Answer from the drawing. Dimensions are ordinates in mm from the lowest x, y and z of the part. Round coordinates to 2 decimals unless told otherwise and drop trailing zeros. Write each loop counter-clockwise with the first axis right and the second up, starting at its lowest first coordinate (ties: lowest second). Pieces come first, ordered by that corner, then holes. Notation, with made-up numbers: (44, -15.75) -> (89, -15.75) arc R3 cw to (89, -10.75) -> close; hole circle Ø1 at (81.5, 62). An arc over 180 degrees is marked (long way). Answer as a JSON object with one key per item and string values. Group by question number.
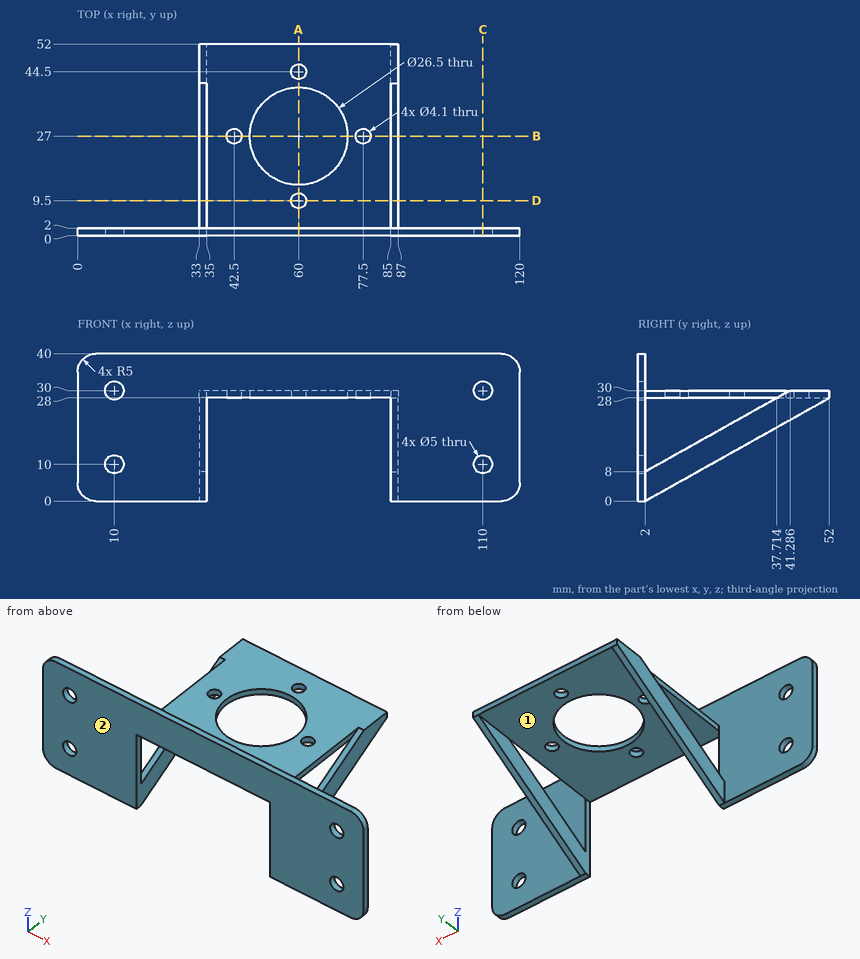
1) A cutting plane is placed at B-B on y = 27. Determine the outline of the cut face in (x, z).
2) Each of these flat-tipped pins is pushed along its axis until it touches: P1, Ø25, axis at x = 49, y = 29.5, coming from the +Z side; P2, Ø6, axis at y = 29, z = 29.5, coming from the +X side; P3, Ø22.5, axis at y = 31, z = 16, coming from the +X side; P4, Ø3.5, axis at x = 42.5, y = 27, coming from the +Z side. Where does it stop, or does it pass through?
3) Straight lines are drawn through the part: L1, parallel to X at y = 0.8, z = 10; L2, parallel to X at y = 0.5, z = 30; L3, parallel to Y at x = 42.5, z = 29.25. For each, find the intervals that lie inside material, in ascending order.
4) A cutting plane is placed at C-C on x = 110. Determine the outline of the cut face in (y, z), plus the area to 3 significant figures.
5) A cutting plane is placed at D-D on y = 9.5. Determine the outline of the cut face in (x, z).
6) A cutting plane is placed at A-A on x = 60. Determine the outline of the cut face in (y, z).
7) For a pull along X with two mould halves and no side action, classify the marked faces 1 and 2 as released by +X, released by -X, zero draft, split by the parting line, or undercut.
Established:
{
 "1": {"outline": "(33, 14) -> (35, 14) -> (35, 22) -> (33, 22) -> close; (35, 28) -> (40.45, 28) -> (40.45, 30) -> (35, 30) -> close; (44.55, 28) -> (46.75, 28) -> (46.75, 30) -> (44.55, 30) -> close; (73.25, 28) -> (75.45, 28) -> (75.45, 30) -> (73.25, 30) -> close; (79.55, 28) -> (85, 28) -> (85, 30) -> (79.55, 30) -> close; (85, 14) -> (87, 14) -> (87, 22) -> (85, 22) -> close"},
 "2": {"P1": "stops at z = 30", "P2": "stops at x = 85", "P3": "stops at x = 87", "P4": "passes through"},
 "3": {"L1": "x = 0 to 7.5, 12.5 to 35, 85 to 107.5, 112.5 to 120", "L2": "x = 0 to 7.5, 12.5 to 107.5, 112.5 to 120", "L3": "y = 0 to 24.95, 29.05 to 52"},
 "4": {"outline": "(0, 0) -> (2, 0) -> (2, 7.5) -> (0, 7.5) -> close; (0, 12.5) -> (2, 12.5) -> (2, 27.5) -> (0, 27.5) -> close; (0, 32.5) -> (2, 32.5) -> (2, 40) -> (0, 40) -> close", "area": "60.0 mm²"},
 "5": {"outline": "(33, 4.2) -> (35, 4.2) -> (35, 12.2) -> (33, 12.2) -> close; (35, 28) -> (57.95, 28) -> (57.95, 30) -> (35, 30) -> close; (62.05, 28) -> (85, 28) -> (85, 30) -> (62.05, 30) -> close; (85, 4.2) -> (87, 4.2) -> (87, 12.2) -> (85, 12.2) -> close"},
 "6": {"outline": "(0, 28) -> (7.45, 28) -> (7.45, 30) -> (2, 30) -> (2, 40) -> (0, 40) -> close; (11.55, 28) -> (13.75, 28) -> (13.75, 30) -> (11.55, 30) -> close; (40.25, 28) -> (42.45, 28) -> (42.45, 30) -> (40.25, 30) -> close; (46.55, 28) -> (52, 28) -> (52, 30) -> (46.55, 30) -> close"},
 "7": {"face 1": "undercut", "face 2": "zero draft"}
}
